Input: part model. Units: mm. Frame: model coordinates. A direction names the side the tool comes from. Give positions to 0.01 mm unless a question says otherwise; leave off trailing zeros. Order: outer loops, then holes, each group sorted by start corner. A loop starts at its lowest first (then second) coordinate and runs counter-clockwise, first axis right, second up. Notation, with made-up numbers: (75.5, -1.5) -> (119.5, -1.5) arc R22 ccw to (119.5, 36.5) -> close; hole circle Ø2 at (78.5, 28). An arc over 180 degrees is marked (long way). Use a Markdown table: item, result. Add a question column.
from build123d import *

# Parameters (mm, degrees)
SKETCH1_W           = 50.8
SKETCH1_H           = 50.8
BOSS_EXTRUDE1_DEPTH = 7.62
SKETCH3_R           = 2.54
CUT_EXTRUDE1_DEPTH  = 6.35
SKETCH4_R           = 6.35
CUT_EXTRUDE2_DEPTH  = 3.175
SKETCH5_R           = 3.175
CUT_EXTRUDE3_DEPTH  = 3.175
SKETCH6_R           = 3.175
CUT_EXTRUDE4_DEPTH  = 3.175
CUT_EXTRUDE5_START  = -3.175
SKETCH7_R           = 3.175
CUT_EXTRUDE5_DEPTH  = 3.175
CUT_EXTRUDE6_START  = -3.175
SKETCH8_R           = 3.175
CUT_EXTRUDE6_DEPTH  = 3.175


with BuildPart() as part:
    # Sketch1 → Boss-Extrude1 (new body)
    with BuildSketch(Plane.XY):
        with Locations((4.049275362, 0.552173913)):
            Rectangle(SKETCH1_W, SKETCH1_H)
    extrude(amount=BOSS_EXTRUDE1_DEPTH)

    # Sketch3 → Cut-Extrude1 (cut)
    with BuildSketch(Plane.XY.offset(7.62)):
        with Locations((-8.650724638, 0.552173913)):
            Circle(SKETCH3_R)
        with Locations((4.049275362, 13.252173913)):
            Circle(SKETCH3_R)
        with Locations((4.049275362, -12.147826087)):
            Circle(SKETCH3_R)
        with Locations((16.749275362, 0.552173913)):
            Circle(SKETCH3_R)
    extrude(amount=-CUT_EXTRUDE1_DEPTH, mode=Mode.SUBTRACT)

    # Sketch4 → Cut-Extrude2 (cut)
    with BuildSketch(Plane.XY.offset(7.62)):
        with Locations((-8.650724638, 13.252173913)):
            Circle(SKETCH4_R)
        with Locations((16.749275362, 13.252173913)):
            Circle(SKETCH4_R)
        with Locations((16.749275362, -12.147826087)):
            Circle(SKETCH4_R)
        with Locations((-8.650724638, -12.147826087)):
            Circle(SKETCH4_R)
    extrude(amount=-CUT_EXTRUDE2_DEPTH, mode=Mode.SUBTRACT)

    # Sketch5 → Cut-Extrude3 (cut)
    with BuildSketch(Plane(origin=(29.449275362, 0, 0), x_dir=(0, 0, -1), z_dir=(1, 0, 0))):
        with Locations(Location((-3.81, 13.252173913, 0), (0, 0, 90))):
            Circle(SKETCH5_R)
        with Locations(Location((-3.81, -12.147826087, 0), (0, 0, 90))):
            Circle(SKETCH5_R)
    extrude(amount=-CUT_EXTRUDE3_DEPTH, mode=Mode.SUBTRACT)

    # Sketch6 → Cut-Extrude4 (cut)
    with BuildSketch(Plane(origin=(0, -24.847826087, 0), x_dir=(-1, 0, 0), z_dir=(0, -1, 0))):
        with Locations(Location((8.650724638, -3.81, 0), (0, 0, 90))):
            Circle(SKETCH6_R)
        with Locations(Location((-16.749275362, -3.81, 0), (0, 0, 90))):
            Circle(SKETCH6_R)
    extrude(amount=-CUT_EXTRUDE4_DEPTH, mode=Mode.SUBTRACT)

    # Sketch7 → Cut-Extrude5 (cut)
    with BuildSketch(Plane.ZY.offset(21.350724638).offset(CUT_EXTRUDE5_START)):
        with Locations(Location((3.81, 13.252173913, 0), (0, 0, 90))):
            Circle(SKETCH7_R)
        with Locations(Location((3.81, -12.147826087, 0), (0, 0, 90))):
            Circle(SKETCH7_R)
    extrude(amount=CUT_EXTRUDE5_DEPTH, mode=Mode.SUBTRACT)

    # Sketch8 → Cut-Extrude6 (cut)
    with BuildSketch(Plane(origin=(0, 25.952173913, 0), x_dir=(1, 0, 0), z_dir=(0, 1, 0)).offset(CUT_EXTRUDE6_START)):
        with Locations(Location((-8.650724638, -3.81, 0), (0, 0, 90))):
            Circle(SKETCH8_R)
        with Locations(Location((16.749275362, -3.81, 0), (0, 0, 90))):
            Circle(SKETCH8_R)
    extrude(amount=CUT_EXTRUDE6_DEPTH, mode=Mode.SUBTRACT)


solid = part.part
Q1. Section query C-C (x = -3). Return loops of the section in (y, z) (3 decimals).
Q2. Ray query, line 1 (X direction, y = 23, z = 3.5); line 2 (Y direction, x = -7, z = 7); line 3 (X direction, y = 12, z = 4.5). Return the intervals inside material, ascending.
Q3. Section query A-A (x = 22). Return loops of the section in (y, z) (3 decimals), plus the area to 3 significant figures.
Q4. Section query B-B (z = 3.81). Give the number of separate pieces and of enclosed holes in the cut face, plus the area to 3 significant figures.
Q5. First-contact query: pin 1 (4.5 mm diameter, centred on x = -8.65, y = 0.55, fed in from -Z); pin 2 (3 mm diameter, centred on x = 4.05, y = 13.25, fed in from +Z); pin 3 (7.5 mm diameter, centred on x = 16.75, y = 13.25, fed in from +Z) (3 decimals); pin 4 (1.9 mm diameter, centred on x = -8, z = 5, fed in from +Y). Flat tips, straight axial feed; report the tip coordinate or a pass-through.
Q6. Access query for faces 5 (the flat face through (-18.176, -12, 4)), 6 (the flat face through (26.274, -12, 4)), 7 (the cylindrical face through (-13.7, -16, 6.1)), 8 (the cylindrical face through (13.6, 24.3, 4.2)). Directions: +Z, -Z, +X, -X, +Y, -Y. A direction counts if a zero-diameter tool reaches every point of the face in a straight line with its end or side. Return the directions, or none.
Q7. Draft query along X for faces 1 (the cylindrical face through (-19.741, -9.215, 5.026)), 2 (the flat face through (17, -21.673, 4)), 3 (the cylindrical face through (14.82, -23.28, 6.33)), 4 (the flat face through (29.449, 0, 4)). Return one class per face: +X half, -X half, draft (parallel to the pull), parting line (faces both ways), or undercut.
Solution:
| question | item | result |
|---|---|---|
| 1 | outline | (-24.848, 0) -> (25.952, 0) -> (25.952, 7.62) -> (16.149, 7.62) -> (16.149, 4.445) -> (10.355, 4.445) -> (10.355, 7.62) -> (-9.251, 7.62) -> (-9.251, 4.445) -> (-15.045, 4.445) -> (-15.045, 7.62) -> (-24.848, 7.62) -> close |
| 2 | line 1 | x = -21.35 to -11.81, -5.49 to 13.59, 19.91 to 29.45 |
| 2 | line 2 | y = -24.85 to -18.28, -6.02 to -1.38, 2.48 to 7.12, 19.38 to 25.95 |
| 2 | line 3 | x = -18.18 to -14.88, -2.43 to 1.84, 6.26 to 10.52, 22.97 to 26.27 |
| 3 | outline | (-24.848, 0) -> (25.952, 0) -> (25.952, 7.62) -> (16.823, 7.62) -> (16.823, 4.445) -> (9.681, 4.445) -> (9.681, 7.62) -> (-8.577, 7.62) -> (-8.577, 4.445) -> (-15.719, 4.445) -> (-15.719, 7.62) -> (-24.848, 7.62) -> close |
| 3 | area | 342 mm² |
| 4 | separate pieces | 1 |
| 4 | enclosed holes | 4 |
| 4 | area | 2,340 mm² |
| 5 | pin 1 | stops at z = 0 |
| 5 | pin 2 | stops at z = 1.27 |
| 5 | pin 3 | stops at z = 4.445 |
| 5 | pin 4 | stops at y = 22.78 |
| 6 | face 5 | -X |
| 6 | face 6 | +X |
| 6 | face 7 | +Z |
| 6 | face 8 | +Y |
| 7 | face 1 | draft |
| 7 | face 2 | undercut |
| 7 | face 3 | undercut |
| 7 | face 4 | +X half |
